Input: part model. Units: mm. Frame: model coordinates. Coordinates: 2 decimals unless noted, no trailing zeros. Order: outer loops, then holes, each group sorted by start corner. A loop starts at its lowest first (then second) coordinate and runs counter-clockwise, first axis right, second up. Notation, with made-up numbers: (-7.5, -19.5) -> (32.5, -19.5) arc R10 cw to (32.5, -6.5) -> close; hole circle Ø6 at (47.5, -10). An arc over 180 degrees is marked (long way). Use one line per item in the form item = value. Start each with the question number.
1) Section query A-A on y = 40.5. Output: boundary loops of the cut face in (x, z), then the cut area to 3 significant figures.
2) Section query D-D on x = 165.5. Output: boundary loops of the cut face in (y, z).
3) Ray query, line 1 along Y through (x, z) = (0, 3); line 2 along Y through (x, z) = (224, 2.2); line 3 along X through (y, z) = (-257.5, 2.2). Return the intervals inside material, ascending.
4) Section query B-B on x = -43. Output: boundary loops of the cut face in (y, z).
5) Section query C-C on z = 2.8. Count the separate pieces of the cut face and the enclosed holes in it, then the cut area to 3 significant figures.
6) Pin query (flat end, axial travel): pin 1 (2 mm diameter, centred on y = -288, z = 2, fed in from -X); pin 2 (2 mm diameter, centred on x = -31, z = 1, fed in from +Y). Return the tip coordinate at first contact, or that it passes through.
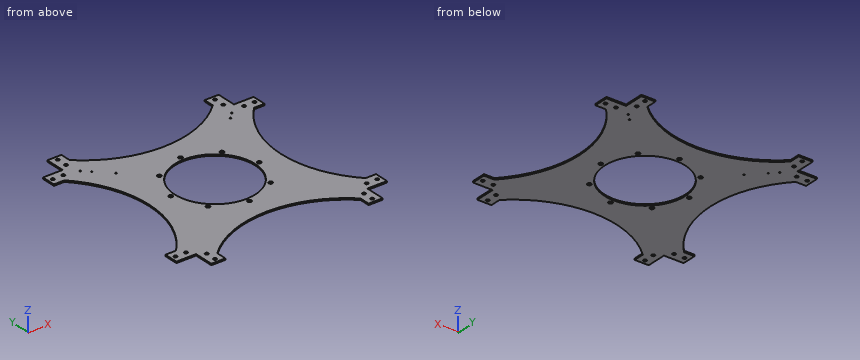
from build123d import *

# Parameters (mm, degrees)
SKETCH1_R          = 114.5
BASE_FLANGE1_DEPTH = 4
SKETCH2_R          = 4.6
EXTRUDE1_DEPTH     = 4
SKETCH3_R          = 5.5
EXTRUDE2_DEPTH     = 4
CIRPATTERN1_COUNT  = 8
SKETCH4_R          = 2.1
CUT_EXTRUDE1_DEPTH = 10


# Sheet-metal steps are written as plain solids
with BuildPart() as part:
    # Sketch1 → Base-Flange1 (new body)
    with BuildSketch(Plane.XY):
        with BuildLine():
            Line((244, 244), (244, 300))
            Line((244, 300), (204, 300))
            Line((204, 300), (204, 270))
            ThreePointArc((204, 270), (0, 188.093876027), (-204, 270))
            Line((-204, 270), (-204, 300))
            Line((-204, 300), (-244, 300))
            Line((-244, 300), (-244, 244))
            Line((-244, 244), (-300, 244))
            Line((-300, 244), (-300, 204))
            Line((-300, 204), (-270, 204))
            ThreePointArc((-270, 204), (-188.093876027, 0), (-270, -204))
            Line((-270, -204), (-300, -204))
            Line((-300, -204), (-300, -244))
            Line((-300, -244), (-244, -244))
            Line((-244, -244), (-244, -300))
            Line((-244, -300), (-204, -300))
            Line((-204, -300), (-204, -270))
            ThreePointArc((-204, -270), (0, -188.093876027), (204, -270))
            Line((204, -270), (204, -300))
            Line((204, -300), (244, -300))
            Line((244, -300), (244, -244))
            Line((244, -244), (300, -244))
            Line((300, -244), (300, -204))
            Line((300, -204), (270, -204))
            ThreePointArc((270, -204), (188.093876027, 0), (270, 204))
            Line((270, 204), (300, 204))
            Line((300, 204), (300, 244))
            Line((300, 244), (244, 244))
        make_face()
        Circle(SKETCH1_R, mode=Mode.SUBTRACT)
    extrude(amount=BASE_FLANGE1_DEPTH)

    # Sketch2 → Extrude1 (cut)
    with BuildSketch(Plane.XY.offset(4)):
        with Locations((224, 287.5)):
            Circle(SKETCH2_R)
        with Locations((224, 257.5)):
            Circle(SKETCH2_R)
        with Locations((257.5, 224)):
            Circle(SKETCH2_R)
        with Locations((287.5, 224)):
            Circle(SKETCH2_R)
        with Locations(Location((287.5, -224, 0), (0, 0, 180))):
            Circle(SKETCH2_R)
        with Locations(Location((257.5, -224, 0), (0, 0, 180))):
            Circle(SKETCH2_R)
        with Locations(Location((224, -257.5, 0), (0, 0, 180))):
            Circle(SKETCH2_R)
        with Locations(Location((224, -287.5, 0), (0, 0, 180))):
            Circle(SKETCH2_R)
        with Locations((-224, -287.5)):
            Circle(SKETCH2_R)
        with Locations((-224, -257.5)):
            Circle(SKETCH2_R)
        with Locations((-257.5, -224)):
            Circle(SKETCH2_R)
        with Locations((-287.5, -224)):
            Circle(SKETCH2_R)
        with Locations(Location((-287.5, 224, 0), (0, 0, 180))):
            Circle(SKETCH2_R)
        with Locations(Location((-257.5, 224, 0), (0, 0, 180))):
            Circle(SKETCH2_R)
        with Locations(Location((-224, 257.5, 0), (0, 0, 180))):
            Circle(SKETCH2_R)
        with Locations(Location((-224, 287.5, 0), (0, 0, 180))):
            Circle(SKETCH2_R)
    extrude(amount=-EXTRUDE1_DEPTH, mode=Mode.SUBTRACT)

    # Sketch3 → Extrude2 (cut)
    with BuildSketch(Plane.XY.offset(4)):
        with Locations((0, 126)):
            Circle(SKETCH3_R)
    extrude2 = extrude(amount=-EXTRUDE2_DEPTH, mode=Mode.SUBTRACT)

    # CirPattern1: Extrude2 ×8 about axis
    cirpattern1_axis = Axis((0, 0, 0), (0, 0, 1))
    for i in range(1, CIRPATTERN1_COUNT):
        add(extrude2.rotate(cirpattern1_axis, i * 360 / CIRPATTERN1_COUNT), mode=Mode.SUBTRACT)

    # Sketch4 → Cut-Extrude1 (cut)
    with BuildSketch(Plane.XY.offset(4)):
        with Locations((215.715728753, 215.715728753)):
            Circle(SKETCH4_R)
        with Locations((199.452272785, 199.452272785)):
            Circle(SKETCH4_R)
        with Locations((-158.440079476, 158.440079476)):
            Circle(SKETCH4_R)
        with Locations((-215.715728753, 215.715728753)):
            Circle(SKETCH4_R)
        with Locations((-197.330952442, 197.330952442)):
            Circle(SKETCH4_R)
    extrude(amount=-CUT_EXTRUDE1_DEPTH, mode=Mode.SUBTRACT)


solid = part.part
Answers below:
q1.outline = (-190.89, 0) -> (-107.1, 0) -> (-107.1, 4) -> (-190.89, 4) -> close; (107.1, 0) -> (190.89, 0) -> (190.89, 4) -> (107.1, 4) -> close
q1.area = 670 mm^2
q2.outline = (-238.89, 0) -> (238.89, 0) -> (238.89, 4) -> (-238.89, 4) -> close
q3.line_1 = -188.09 to -131.5, -120.5 to -114.5, 114.5 to 120.5, 131.5 to 188.09
q3.line_2 = -300 to -292.1, -282.9 to -262.1, -252.9 to -141.05, 141.05 to 252.9, 262.1 to 282.9, 292.1 to 300
q3.line_3 = -244 to -228.6, -219.4 to -190.09, 190.09 to 219.4, 228.6 to 244
q4.outline = (-191.24, 0) -> (-106.12, 0) -> (-106.12, 4) -> (-191.24, 4) -> close; (106.12, 0) -> (191.24, 0) -> (191.24, 4) -> (106.12, 4) -> close
q5.separate_pieces = 1
q5.enclosed_holes = 30
q5.area = 163,000 mm^2
q6.pin_1 = -244
q6.pin_2 = 189.83
